```python
from build123d import *

# Parameters (mm, degrees)
BOSS_EXTRUDE1_DEPTH = 5
SKETCH2_W           = 4
SKETCH2_H           = 10
CUT_EXTRUDE1_DEPTH  = 10
SKETCH3_R           = 6
SKETCH3_W           = 4
SKETCH3_H           = 10
CUT_EXTRUDE2_DEPTH  = 10


with BuildPart() as part:
    # Sketch1 → Boss-Extrude1 (new body)
    with BuildSketch(Plane.XY):
        with BuildLine():
            Line((-165, 125), (165, 125))
            ThreePointArc((165, 125), (172.071067812, 122.071067812), (175, 115))
            Line((175, 115), (175, -115))
            ThreePointArc((175, -115), (172.071067812, -122.071067812), (165, -125))
            Line((165, -125), (-165, -125))
            ThreePointArc((-165, -125), (-172.071067812, -122.071067812), (-175, -115))
            Line((-175, -115), (-175, 115))
            ThreePointArc((-175, 115), (-172.071067812, 122.071067812), (-165, 125))
        make_face()
    extrude(amount=BOSS_EXTRUDE1_DEPTH)

    # Sketch2 → Cut-Extrude1 (cut)
    with BuildSketch(Plane.XY.offset(5)):
        with Locations((99.328502067, 111.512009489)):
            Rectangle(SKETCH2_W, SKETCH2_H)
        with Locations((99.262510454, 72.917517572)):
            Rectangle(SKETCH2_W, SKETCH2_H)
        with Locations((58.394493679, 72.917517572)):
            Rectangle(SKETCH2_W, SKETCH2_H)
        with Locations((58.328502067, 111.512009489)):
            Rectangle(SKETCH2_W, SKETCH2_H)
        with Locations((58.328502067, -111.512009489)):
            Rectangle(SKETCH2_W, SKETCH2_H)
        with Locations((58.394493679, -72.917517572)):
            Rectangle(SKETCH2_W, SKETCH2_H)
        with Locations((99.262510454, -72.917517572)):
            Rectangle(SKETCH2_W, SKETCH2_H)
        with Locations((99.328502067, -111.512009489)):
            Rectangle(SKETCH2_W, SKETCH2_H)
        with Locations((-99.328502067, -111.512009489)):
            Rectangle(SKETCH2_W, SKETCH2_H)
        with Locations((-99.262510454, -72.917517572)):
            Rectangle(SKETCH2_W, SKETCH2_H)
        with Locations((-58.394493679, -72.917517572)):
            Rectangle(SKETCH2_W, SKETCH2_H)
        with Locations((-58.328502067, -111.512009489)):
            Rectangle(SKETCH2_W, SKETCH2_H)
        with Locations((-58.328502067, 111.512009489)):
            Rectangle(SKETCH2_W, SKETCH2_H)
        with Locations((-58.394493679, 72.917517572)):
            Rectangle(SKETCH2_W, SKETCH2_H)
        with Locations((-99.262510454, 72.917517572)):
            Rectangle(SKETCH2_W, SKETCH2_H)
        with Locations((-99.328502067, 111.512009489)):
            Rectangle(SKETCH2_W, SKETCH2_H)
    extrude(amount=-CUT_EXTRUDE1_DEPTH, mode=Mode.SUBTRACT)

    # Sketch3 → Cut-Extrude2 (cut)
    with BuildSketch(Plane.XY.offset(5)):
        with Locations((-115, 0)):
            Circle(SKETCH3_R)
        with Locations((162, 0)):
            Rectangle(SKETCH3_W, SKETCH3_H)
        with Locations((64, 0)):
            Rectangle(SKETCH3_W, SKETCH3_H)
    extrude(amount=-CUT_EXTRUDE2_DEPTH, mode=Mode.SUBTRACT)


solid = part.part
```
Read the model definition and answer for the solid it produces. Units are mm, in the model's axes. Give positions to 0.01 mm unless a question says otherwise; leave off trailing zeros. Write each loop counter-clockwise with the first axis right and the second up, starting at its lowest first coordinate (ties: lowest second). Pieces come first, ordered by that corner, then holes. Notation, with made-up numbers: (5.5, -12.5) - (43.5, -12.5) arc R20 cw to (43.5, 3.5) - close; hole circle Ø10 at (-33, 1.25). An arc over 180 degrees is marked (long way). Write item = value, one per line. Start each with the question number.
Item 1: Find section A-A (y = 73). Give the vertices of the cut face in (x, z).
Item 2: Find section B-B (x = -115). Give the vertices of the cut face in (y, z), then the cut area to 3 significant figures.
Item 3: Find section C-C (y = 0). Give the vertices of the cut face in (x, z), then the cut area to 3 significant figures.
Item 4: Find the intervals of material crossed by probe 1 along X at (y, z) = (1, 1.7); probe 2 along X at (y, z) = (71, 3.7); probe 3 along Y at (x, z) = (-115, 3.8), in increasing order. Write a range as [from, to].
Item 5: The mould has two halves that part along Y. Classify faces 1 (the flat face through (2, 2, 0)), 2 (the cylindrical face through (-121, 0, 3)), 3 (the cylindrical face through (-172.15, 121.99, 2.46)), 4 (the cylindrical face through (-171.99, -122.15, 2.46)): +Y half, -Y half, draft (parallel to the pull), parting line (faces both ways), or undercut.
Response:
q1.outline = (-175, 0) - (-101.26, 0) - (-101.26, 5) - (-175, 5) - close; (-97.26, 0) - (-60.39, 0) - (-60.39, 5) - (-97.26, 5) - close; (-56.39, 0) - (56.39, 0) - (56.39, 5) - (-56.39, 5) - close; (60.39, 0) - (97.26, 0) - (97.26, 5) - (60.39, 5) - close; (101.26, 0) - (175, 0) - (175, 5) - (101.26, 5) - close
q2.outline = (-125, 0) - (-6, 0) - (-6, 5) - (-125, 5) - close; (6, 0) - (125, 0) - (125, 5) - (6, 5) - close
q2.area = 1,190 mm²
q3.outline = (-175, 0) - (-121, 0) - (-121, 5) - (-175, 5) - close; (-109, 0) - (62, 0) - (62, 5) - (-109, 5) - close; (66, 0) - (160, 0) - (160, 5) - (66, 5) - close; (164, 0) - (175, 0) - (175, 5) - (164, 5) - close
q3.area = 1,650 mm²
q4.probe_1 = [-175, -120.92], [-109.08, 62], [66, 160], [164, 175]
q4.probe_2 = [-175, -101.26], [-97.26, -60.39], [-56.39, 56.39], [60.39, 97.26], [101.26, 175]
q4.probe_3 = [-125, -6], [6, 125]
q5.face_1 = draft
q5.face_2 = undercut
q5.face_3 = +Y half
q5.face_4 = -Y half
